The model under review builds one solid part; all positions refer to its coordinate system, in mm. A direction names the side the tool comes from. Round coordinates to 2 decimals unless told otherwise and drop trailing zeros. Loops run counter-clockwise (first coordinate to the right, second up) from the corner with the lowest first, then second, coordinate; pieces in that order, holes last. Notation, with made-up numbers: M 63.25,16.25 L 88.25,16.25 A23 cw 88.25,54.25 Z; hole C -38.75,45 d9. An arc over 180 degrees is marked long. Answer as a JSON object with one key per item and string values. Group by question number.
Item 1: Consider section D-D (z = 2). Give the boundary of the cut face in (x, y), and give its area (3 significant figures).
Item 2: Tool access review of faces 4 (the face through (6.35, 0, 18)), 5 (the face through (3, 9, 25.4)), 6 (the face through (3, 6.35, 22)), 7 (the face through (38.1, 0, 6)): name each direction out of +Z, -Z, +X, -X, +Y, -Y from which nothing blocks a thin tool from reaching the whole face with its end or side.
Item 3: Consider section C-C (y = 1.75). Give the boundary of the cut face in (x, z).
Item 4: To check wall thickness, follow line 1 (Y direction, x = 49, z = 4.5); line 2 (X direction, y = 4.25, z = 14.25). State the ranges of each line that lie inside material, in increasing order.
Item 5: The part is to be moulded in two halves that separate along Y. For faces 1 (the face through (3, -6.35, 22)), 2 (the face through (24, 0, 12.7)), 3 (the face through (25, 12.7, 7)), say which applies: +Y half, -Y half, draft (parallel to the pull), parting line (faces both ways), or undercut.
Item 6: Consider section A-A (z = 22.5). Give the boundary of the cut face in (x, y), and give its area (3 significant figures).
Item 7: Consider section B-B (x = 4). Give the boundary of the cut face in (y, z), and give its area (3 significant figures).
Item 8: Insertion check: P1, Ø4, axis at y = -7, z = 14, coming from the -X side; P2, Ø2, axis at y = 1.5, z = 7.5, coming from the +X side; P3, Ø7.5, axis at x = 26.5, y = 2.5, coming from the +Z side; P4, Ø4, axis at y = -0.5, z = 17.5, coming from the +X side. Each pin has a flat end and moves straight along its axis. Give the tip position at first contact, or say it passes through.
```python
from build123d import *

# Parameters (mm, degrees)
F1_DEPTH = 12.7
F2_W     = 6.35
F2_H     = 12.7
F3_DEPTH = 6.35
F4_W     = 12.7
F4_H     = 12.7
F5_DEPTH = 12.701


with BuildPart() as f1:
    # F0 (on Front) → F1 (new body, symmetric)
    with BuildSketch(Plane.XZ):
        Polygon((0, 25.4), (0, 0), (50.8, 0), (50.8, 12.7), (6.35, 12.7), (6.35, 25.4), align=None)
    extrude(amount=F1_DEPTH, both=True)

    # F2 (on face) → F3 (cut)
    with BuildSketch(Plane.XY.offset(25.4)):
        with Locations((3.175, 0)):
            Rectangle(F2_W, F2_H)
    extrude(amount=-F3_DEPTH, mode=Mode.SUBTRACT)

    # F4 (on face) → F5 (cut, through all)
    with BuildSketch(Plane.XY.offset(12.7)):
        with Locations((44.45, 0)):
            Rectangle(F4_W, F4_H)
    extrude(amount=-F5_DEPTH, mode=Mode.SUBTRACT)


solid = f1.part
```
Geometry results:
{
 "1": {"outline": "M 0,-12.7 L 50.8,-12.7 L 50.8,-6.35 L 38.1,-6.35 L 38.1,6.35 L 50.8,6.35 L 50.8,12.7 L 0,12.7 Z", "area": "1,130 mm^2"},
 "2": {"face 4": "+Z, +X, +Y, -Y", "face 5": "+Z, +X, -X, +Y, -Y", "face 6": "+Z, +X, -X", "face 7": "+Z, -Z, +X"},
 "3": {"outline": "M 0,0 L 38.1,0 L 38.1,12.7 L 6.35,12.7 L 6.35,19.05 L 0,19.05 Z"},
 "4": {"line 1": "y = -12.7 to -6.35, 6.35 to 12.7", "line 2": "x = 0 to 6.35"},
 "5": {"face 1": "undercut", "face 2": "draft", "face 3": "+Y half"},
 "6": {"outline": "M 0,-12.7 L 6.35,-12.7 L 6.35,-6.35 L 0,-6.35 Z; M 0,6.35 L 6.35,6.35 L 6.35,12.7 L 0,12.7 Z", "area": "80.6 mm^2"},
 "7": {"outline": "M -12.7,0 L 12.7,0 L 12.7,25.4 L 6.35,25.4 L 6.35,19.05 L -6.35,19.05 L -6.35,25.4 L -12.7,25.4 Z", "area": "565 mm^2"},
 "8": {"P1": "stops at x = 0", "P2": "stops at x = 38.1", "P3": "stops at z = 12.7", "P4": "stops at x = 6.35"}
}
